Check sheet for the modelled part. Datum: model origin and axes. Units: mm. A direction names the side the tool comes from. Round coordinates to 2 decimals unless told otherwise and drop trailing zeros. Write each loop counter-clockwise with the first axis right and the second up, starting at its lowest first coordinate (ties: lowest second). Pieces come first, ordered by that corner, then holes.
Item 1: Section check B-B, the plane z = 0. Record the cut outline in (x, y) (3 decimals), plus the area to 3 significant figures.
Item 2: Release check for a two-part mould opening along X. For faces 1 (the flat face through (59.912, 38, 0)), 2 (the flat face through (59.34, 24.79, -25)), 3 (the flat face through (59.175, 38, 0)) record: pulls with the +X half, pulls with the -X half, needs draft (parallel to the pull), parting line crosses it, or undercut.
Item 3: Section check C-C, the plane y = 8. Record the cut outline in (x, z) (3 decimals), plus the area to 3 significant figures.
Item 4: Section check D-D, the plane z = -18.5. Record the cut outline in (x, y) (3 decimals).
Item 5: Section check A-A, the plane x = 55.75. Record the cut outline in (y, z).
Item 6: Material ranges on line 1 along X through (y, z) = (60.5, 22.5) (3 decimals); line 2 along Y through (x, z) = (50.5, -0.5); line 3 along Y through (x, z) = (52, -21), recorded low to high.
Item 7: Depth check by flat-ended pin: pin 1 (3.5 mm diameter, centred on x = 54.5, z = 19, fed in from +Y); pin 2 (4 mm diameter, centred on y = 12.5, z = 11, fed in from +X). Enter the tip coordinate at first touch or a pass-through.
Item 8: Set-up check for faces 4 (the flat face through (50.6, 25, 25)), 5 (the flat face through (50.6, 6.2, -11.25)), 6 (the flat face through (55, 0, 18)): record each of +Z, -Z, +X, -X, +Y, -Y from which the full face is reachable in a straight line by a thin tool's end or side.
from build123d import *

# Parameters (mm, degrees)
SKETCH2_W                  = 40
SKETCH2_H                  = 22.5
BASE_FLANGE1_DEPTH         = 0.7366
SKETCHED_START             = -25
SKETCHED_BEND1_DEPTH       = 50
SKETCHED_BEND1_2_DEPTH     = 13.75
SKETCHED_START_2           = 11.25
SKETCHED_BEND1_3_DEPTH     = 13.75
SKETCHED_START_3           = -26
SKETCHED_BEND1_4_OUTLINE_W = 0.7366
SKETCHED_BEND1_4_OUTLINE_H = 50
SKETCHED_BEND1_4_DEPTH     = 61
SKETCHED_START_4           = 75
SKETCHED_BEND1_5_OUTLINE_W = 0.7366
SKETCHED_BEND1_5_OUTLINE_H = 50
SKETCHED_BEND1_5_DEPTH     = 61
SKETCHED_START_5           = 50.0884
SKETCHED_BEND1_6_DEPTH     = 0.7366
SKETCHED_START_6           = 59.175
SKETCHED_BEND1_7_DEPTH     = 0.7366


with BuildPart() as part:
    # Base-Flange1: sheet metal written as solids
    # Sketch2 → Base-Flange1 (new body)
    with BuildSketch(Plane(origin=(0, 0, 0), x_dir=(1, 0, 0), z_dir=(0, 1, 0))):
        with BuildLine():
            Line((0, 25), (110, 25))
            ThreePointArc((110, 25), (135, 0), (110, -25))
            Line((110, -25), (0, -25))
            ThreePointArc((0, -25), (-25, 0), (0, 25))
        make_face()
        with Locations((55, 0)):
            Rectangle(SKETCH2_W, SKETCH2_H, mode=Mode.SUBTRACT)
    extrude(amount=-BASE_FLANGE1_DEPTH)

    # Sketched Bend1: read off the stored shape, not the designer's step
    # Sketched Bend1 outline → Sketched Bend1 (cut)
    with BuildSketch(Plane.XY.offset(SKETCHED_START)):
        with BuildLine():
            Line((35, -0.7366), (51.5616, -0.7366))
            ThreePointArc((51.5616, -0.7366), (50.825, -0.539228625), (50.285771375, 0))
            Line((50.285771375, 0), (35, 0))
            Line((35, 0), (35, -0.7366))
        make_face()
        with BuildLine():
            ThreePointArc((59.714228625, 0), (59.175, -0.539228625), (58.4384, -0.7366))
            Line((58.4384, -0.7366), (75, -0.7366))
            Line((75, -0.7366), (75, 0))
            Line((75, 0), (59.714228625, 0))
        make_face()
    extrude(amount=SKETCHED_BEND1_DEPTH, mode=Mode.SUBTRACT)

    # Sketched Bend1 2 outline → Sketched Bend1 2 (add)
    with BuildSketch(Plane.XY.offset(SKETCHED_START)):
        with BuildLine():
            ThreePointArc((50.0884, 0.7366), (50.138598073, 0.355307783), (50.285771375, 0))
            Line((50.285771375, 0), (51.5616, 0))
            ThreePointArc((51.5616, 0), (51.040745145, 0.215745145), (50.825, 0.7366))
            Line((50.825, 0.7366), (50.825, 15.562627139))
            Line((50.825, 15.562627139), (50.0884, 15.562627139))
            Line((50.0884, 15.562627139), (50.0884, 0.7366))
        make_face()
        with BuildLine():
            Line((58.4384, 0), (59.714228625, 0))
            ThreePointArc((59.714228625, 0), (59.861401927, 0.355307783), (59.9116, 0.7366))
            Line((59.9116, 0.7366), (59.9116, 15.562627139))
            Line((59.9116, 15.562627139), (59.175, 15.562627139))
            Line((59.175, 15.562627139), (59.175, 0.7366))
            ThreePointArc((59.175, 0.7366), (58.959254855, 0.215745145), (58.4384, 0))
        make_face()
    extrude(amount=SKETCHED_BEND1_2_DEPTH)

    # Sketched Bend1 3 outline → Sketched Bend1 3 (add)
    with BuildSketch(Plane.XY.offset(SKETCHED_START_2)):
        with BuildLine():
            ThreePointArc((50.0884, 0.7366), (50.138598073, 0.355307783), (50.285771375, 0))
            Line((50.285771375, 0), (51.5616, 0))
            ThreePointArc((51.5616, 0), (51.040745145, 0.215745145), (50.825, 0.7366))
            Line((50.825, 0.7366), (50.825, 15.562627139))
            Line((50.825, 15.562627139), (50.0884, 15.562627139))
            Line((50.0884, 15.562627139), (50.0884, 0.7366))
        make_face()
        with BuildLine():
            Line((58.4384, 0), (59.714228625, 0))
            ThreePointArc((59.714228625, 0), (59.861401927, 0.355307783), (59.9116, 0.7366))
            Line((59.9116, 0.7366), (59.9116, 15.562627139))
            Line((59.9116, 15.562627139), (59.175, 15.562627139))
            Line((59.175, 15.562627139), (59.175, 0.7366))
            ThreePointArc((59.175, 0.7366), (58.959254855, 0.215745145), (58.4384, 0))
        make_face()
    extrude(amount=SKETCHED_BEND1_3_DEPTH)

    # Sketched Bend1 4 outline → Sketched Bend1 4 (cut)
    with BuildSketch(Plane.YZ.offset(SKETCHED_START_3)):
        with Locations((-0.3683, 0)):
            Rectangle(SKETCHED_BEND1_4_OUTLINE_W, SKETCHED_BEND1_4_OUTLINE_H)
    extrude(amount=SKETCHED_BEND1_4_DEPTH, mode=Mode.SUBTRACT)

    # Sketched Bend1 5 outline → Sketched Bend1 5 (cut)
    with BuildSketch(Plane.YZ.offset(SKETCHED_START_4)):
        with Locations((-0.3683, 0)):
            Rectangle(SKETCHED_BEND1_5_OUTLINE_W, SKETCHED_BEND1_5_OUTLINE_H)
    extrude(amount=SKETCHED_BEND1_5_DEPTH, mode=Mode.SUBTRACT)

    # Sketched Bend1 6 outline → Sketched Bend1 6 (add)
    with BuildSketch(Plane.YZ.offset(SKETCHED_START_5)):
        with BuildLine():
            ThreePointArc((50.562627139, -25), (75.562627139, 0), (50.562627139, 25))
            Line((50.562627139, 25), (15.562627139, 25))
            Line((15.562627139, 25), (15.562627139, -25))
            Line((15.562627139, -25), (50.562627139, -25))
        make_face()
    extrude(amount=SKETCHED_BEND1_6_DEPTH)

    # Sketched Bend1 7 outline → Sketched Bend1 7 (add)
    with BuildSketch(Plane.YZ.offset(SKETCHED_START_6)):
        with BuildLine():
            ThreePointArc((50.562627139, -25), (75.562627139, 0), (50.562627139, 25))
            Line((50.562627139, 25), (15.562627139, 25))
            Line((15.562627139, 25), (15.562627139, -25))
            Line((15.562627139, -25), (50.562627139, -25))
        make_face()
    extrude(amount=SKETCHED_BEND1_7_DEPTH)


solid = part.part
Values found:
1. outline: (50.088, 15.563) - (50.825, 15.563) - (50.825, 75.563) - (50.088, 75.563) - close; (59.175, 15.563) - (59.912, 15.563) - (59.912, 75.563) - (59.175, 75.563) - close
1. area: 88.4 mm2
2. face 1: pulls with the +X half
2. face 2: needs draft
2. face 3: undercut
3. outline: (50.088, -25) - (50.825, -25) - (50.825, -11.25) - (50.088, -11.25) - close; (50.088, 11.25) - (50.825, 11.25) - (50.825, 25) - (50.088, 25) - close; (59.175, -25) - (59.912, -25) - (59.912, -11.25) - (59.175, -11.25) - close; (59.175, 11.25) - (59.912, 11.25) - (59.912, 25) - (59.175, 25) - close
3. area: 40.5 mm2
4. outline: (50.088, 0.737) arc R1.473 ccw to (51.562, -0.737) - (58.438, -0.737) arc R1.473 ccw to (59.912, 0.737) - (59.912, 67.378) - (59.175, 67.378) - (59.175, 0.737) arc R0.737 cw to (58.438, 0) - (51.562, 0) arc R0.737 cw to (50.825, 0.737) - (50.825, 67.378) - (50.088, 67.378) - close
5. outline: (-0.74, -25) - (0, -25) - (0, -11.25) - (-0.74, -11.25) - close; (-0.74, 11.25) - (0, 11.25) - (0, 25) - (-0.74, 25) - close
6. line 1: x = 50.088 to 50.825, 59.175 to 59.912
6. line 2: y = 15.56 to 75.56
6. line 3: y = -0.74 to 0
7. pin 1: stops at y = 0
7. pin 2: stops at x = 59.91
8. face 4: +Z, +X, -X, +Y, -Y
8. face 5: +X, -X, -Y
8. face 6: +Z, -Z, +Y
